Autodesk Fusion 360 part; units mm, degrees
sketch "Sketch1" plane through (0, 0, 0) normal (0, 0, 1) x (1, 0, 0)
  line L0 (0, 0) -> (32, 0)
  line L1 (32, 0) -> (32, 39)
  line L2 (32, 39) -> (0, 39)
  line L3 (0, 39) -> (0, 0)
  dimension "d1" = 32
  dimension "d2" = 39
extrude "Extrude1" add sketch "Sketch1" along normal blind 1.6
sketch "Sketch2" plane through (0, 0, 1.6) normal (0, 0, 1) x (-1, 0, 0)
  line L0 (0, -39) -> (0, 0)
  line L1 (0, 0) -> (-32, 0)
  line L2 (-32, 0) -> (-32, -39)
  line L3 (-32, -39) -> (0, -39)
  line L4 (-7.5, -24.3) -> (-24.5, -24.3)
  line L5 (-24.5, -24.3) -> (-24.5, -6.4)
  line L6 (-24.5, -6.4) -> (-7.5, -6.4)
  line L7 (-7.5, -6.4) -> (-7.5, -24.3)
  dimension "d5" = 14.7
  dimension "d6" = 6.4
  dimension "d7" = 7.5
  dimension "d8" = 7.5
extrude "Extrude2" add sketch "Sketch2" along normal blind 3.2 contours L4 L5 L6 L7
sketch "Sketch3" plane through (0, 0, 1.6) normal (0, 0, 1) x (-1, 0, 0)
  line L0 (-7.5, -6.4) -> (-7.5, -24.3)
  line L1 (-7.5, -24.3) -> (-24.5, -24.3)
  line L2 (-24.5, -24.3) -> (-24.5, -6.4)
  line L3 (-24.5, -6.4) -> (-7.5, -6.4)
  line L4 (0, -39) -> (0, 0)
  line L5 (0, 0) -> (-32, 0)
  line L6 (-32, 0) -> (-32, -39)
  line L7 (-32, -39) -> (0, -39)
  line L8 (-11.8, -34.3) -> (-20.2, -34.3)
  line L9 (-20.2, -34.3) -> (-20.2, -40.2)
  line L10 (-20.2, -40.2) -> (-11.8, -40.2)
  line L11 (-11.8, -40.2) -> (-11.8, -34.3)
  dimension "d11" = 11.8
  dimension "d12" = 11.8
  dimension "d14" = 1.2
  dimension "d15" = 4.7
extrude "Extrude3" add sketch "Sketch3" along normal blind 2.6 contours L7 L9 L10 L11 | L7 L8 L9 L11
equation "d9 = 4.8 mm - 1.6 mm"
equation "d16 = 4.2 mm - 1.6 mm"
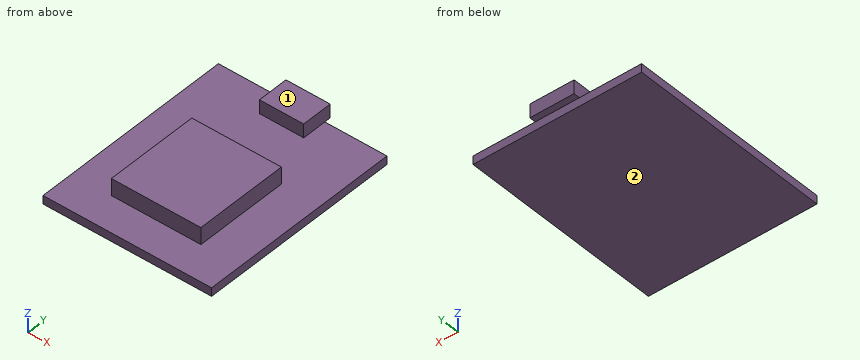
For this review, take the finished solid that the model builds, in its own axes (mm). Face numbers are marked on the shaded views. A direction names the side the tool comes from. Round coordinates to 2 decimals unless told otherwise and drop trailing zeros. Loops run counter-clockwise (first coordinate to the right, second up) from the corner with the lowest first, then second, coordinate; pieces in that order, holes last. Notation, with made-up numbers: (81.5, 29.5) - (104.5, 29.5) arc R21 ccw to (104.5, 39.5) - close; hole circle Ø8 at (15, 22). An arc over 180 degrees is marked (long way). Use one line per item in the form item = value.
1) We need section C-C on x = 17. Write out the cut boundary in (y, z).
Solutions:
outline = (0, 0) - (39, 0) - (39, 1.6) - (40.2, 1.6) - (40.2, 4.2) - (34.3, 4.2) - (34.3, 1.6) - (24.3, 1.6) - (24.3, 4.8) - (6.4, 4.8) - (6.4, 1.6) - (0, 1.6) - close
2) We need section D-D on y = 11. Write out the cut boundary in (x, z), then the cut area to 3 significant figures.
Solutions:
outline = (0, 0) - (32, 0) - (32, 1.6) - (24.5, 1.6) - (24.5, 4.8) - (7.5, 4.8) - (7.5, 1.6) - (0, 1.6) - close
area = 106 mm2
3) We need section B-B on y = 36. Write out the cut boundary in (x, z), then the cut area to 3 significant figures.
Solutions:
outline = (0, 0) - (32, 0) - (32, 1.6) - (20.2, 1.6) - (20.2, 4.2) - (11.8, 4.2) - (11.8, 1.6) - (0, 1.6) - close
area = 73.0 mm2
4) Clearance check with flat-ended pins moving along their axes: P1, Ø1.8, axis at x = 16.5, z = 1, coming from the +Y side; P2, Ø1, axis at x = 26.5, z = 4, coming from the -Y side; P3, Ø6.5, axis at x = 17.5, y = 37.5, coming from the +Z side; P4, Ø1.6, axis at y = 17.5, z = 3.5, coming from the +X side. State where each tip first meets the part, or that it passes through.
Solutions:
P1 = 40.2
P2 = through
P3 = 4.2
P4 = 24.5
5) We need section A-A on z = 3.3. Write out the cut boundary in (x, y), then the cut area to 3 significant figures.
Solutions:
outline = (7.5, 6.4) - (24.5, 6.4) - (24.5, 24.3) - (7.5, 24.3) - close; (11.8, 34.3) - (20.2, 34.3) - (20.2, 40.2) - (11.8, 40.2) - close
area = 354 mm2
6) Tool access review of the marked faces 1 and 2: name each direction out of +Z, -Z, +X, -X, +Y, -Y from which nothing blocks a thin tool from reaching the whole face with its end or side.
Solutions:
face_1 = +Z, +X, -X, +Y
face_2 = -Z, +X, -X, +Y, -Y
7) Wall thickness on probe 1 along Y at (x, z) = (15, 2.75); probe 2 along Z at (x, y) = (30, 18); probe 3 along X at (y, z) = (19, 1.95): over which ranges is each line inside the solid? List them lowest first.
Solutions:
probe_1 = 6.4 to 24.3, 34.3 to 40.2
probe_2 = 0 to 1.6
probe_3 = 7.5 to 24.5
